Model file for the job. Use its own axes, mm. Face numbers are marked on the shaded views. A direction names the side the tool comes from. Round coordinates to 2 decimals unless told otherwise and drop trailing zeros. Loops run counter-clockwise (first coordinate to the right, second up) from the corner with the lowest first, then second, coordinate; pieces in that order, holes last. Notation, with made-up numbers: M -30.75,-24 L -5.75,-24 A17 ccw -5.75,-8 Z; hole C -31.75,-11 d7. An arc over 180 degrees is marked long. Use a Markdown table: item, result. Add a question column.
Q1. Tool access for the marked faces 1 and 2: list every direction of +Z, -Z, +X, -X, +Y, -Y with a clear straight run to the whole face (end or side of a thin tool).
Q2. Cut at A-A (z = 0). Give the cut face in (x, y), plus the area to 3 significant figures.
Q3. Cut at D-D (y = 9.5). Give the cut face in (x, z), plus the area to 3 significant figures.
Q4. Pin check, flat tips, straight feed: pin 1 (3 mm diameter, centred on x = -1.5, y = 1, fed in from +Z); pin 2 (1.2 mm diameter, centred on y = 1, z = -44.5, fed in from +X); pin 3 (3 mm diameter, centred on x = -1.5, y = 1, fed in from -Z). Stop position of each tip, or through.
Q5. Cut at C-C (x = 48.5). Give the cut face in (y, z).
Q6. Cut at B-B (x = -32). Give the cut face in (y, z), plus the area to 3 significant figures.
Q7. Probe line 1 (Z direction, x = 0, y = 78); line 2 (Y direction, x = -3.5, z = 51); line 3 (Z direction, x = 2, y = 65.5). List the from-to ranges inside material, lowest first. Write a range as from..to.
Autodesk Fusion 360 part; units mm, degrees
sketch "Sketch1" plane through (0, 0, 0) normal (0, 1, 0) x (1, 0, 0)
  line L0 (-3, 15) -> (3, 15)
  line L1 (3, 15) -> (3, 55)
  line L2 (3, 55) -> (-3, 55)
  line L3 (-3, 55) -> (-3, 15)
  line L4 (8.8168, 12.1353) -> (11.2438, 10.3719)
  line L5 (8.8168, 12.1353) -> (6.3897, 13.8986)
  line L6 (6.3897, 13.8986) -> (29.9011, 46.2593)
  line L7 (29.9011, 46.2593) -> (34.7552, 42.7326)
  line L8 (34.7552, 42.7326) -> (11.2438, 10.3719)
  line L9 (14.2658, 4.6353) -> (13.3388, 7.4884)
  line L10 (13.3388, 7.4884) -> (15.1929, 1.7821)
  line L11 (15.1929, 1.7821) -> (53.2352, 14.1428)
  line L12 (53.2352, 14.1428) -> (51.3811, 19.8491)
  line L13 (51.3811, 19.8491) -> (13.3388, 7.4884)
  line L14 (14.2658, -4.6353) -> (13.3388, -7.4884)
  line L15 (13.3388, -7.4884) -> (15.1929, -1.7821)
  line L16 (15.1929, -1.7821) -> (53.2352, -14.1428)
  line L17 (53.2352, -14.1428) -> (51.3811, -19.8491)
  line L18 (51.3811, -19.8491) -> (13.3388, -7.4884)
  line L19 (8.8168, -12.1353) -> (11.2438, -10.3719)
  line L20 (11.2438, -10.3719) -> (34.7552, -42.7326)
  line L21 (34.7552, -42.7326) -> (29.9011, -46.2593)
  line L22 (29.9011, -46.2593) -> (6.3897, -13.8986)
  line L23 (6.3897, -13.8986) -> (8.8168, -12.1353)
  line L24 (0, -15) -> (3, -15)
  line L25 (3, -15) -> (-3, -15)
  line L26 (-3, -15) -> (-3, -55)
  line L27 (-3, -55) -> (3, -55)
  line L28 (3, -55) -> (3, -15)
  line L29 (-8.8168, -12.1353) -> (-6.3897, -13.8986)
  line L30 (-6.3897, -13.8986) -> (-11.2438, -10.3719)
  line L31 (-11.2438, -10.3719) -> (-34.7552, -42.7326)
  line L32 (-34.7552, -42.7326) -> (-29.9011, -46.2593)
  line L33 (-29.9011, -46.2593) -> (-6.3897, -13.8986)
  line L34 (-14.2658, -4.6353) -> (-13.3388, -7.4884)
  line L35 (-13.3388, -7.4884) -> (-15.1929, -1.7821)
  line L36 (-15.1929, -1.7821) -> (-53.2352, -14.1428)
  line L37 (-53.2352, -14.1428) -> (-51.3811, -19.8491)
  line L38 (-51.3811, -19.8491) -> (-13.3388, -7.4884)
  line L39 (-14.2658, 4.6353) -> (-13.3388, 7.4884)
  line L40 (-13.3388, 7.4884) -> (-15.1929, 1.7821)
  line L41 (-15.1929, 1.7821) -> (-53.2352, 14.1428)
  line L42 (-53.2352, 14.1428) -> (-51.3811, 19.8491)
  line L43 (-51.3811, 19.8491) -> (-13.3388, 7.4884)
  line L44 (-8.8168, 12.1353) -> (-6.3897, 13.8986)
  line L45 (-6.3897, 13.8986) -> (-11.2438, 10.3719)
  line L46 (-11.2438, 10.3719) -> (-34.7552, 42.7326)
  line L47 (-34.7552, 42.7326) -> (-29.9011, 46.2593)
  line L48 (-29.9011, 46.2593) -> (-6.3897, 13.8986)
  circle A0 centre (0, 0) radius 60
  dimension "d20" = 15
  dimension "d21" = 15
  dimension "d22" = 15
  dimension "d23" = 15
  dimension "d24" = 15
  dimension "d25" = 15
  dimension "d26" = 15
  dimension "d27" = 15
  dimension "d28" = 15
  dimension "d29" = 40
  dimension "d30" = 6
  dimension "d31" = 40
  dimension "d32" = 3
  dimension "d33" = 3
  dimension "d34" = 40
  dimension "d35" = 6
  dimension "d36" = 3
  dimension "d37" = 6
  dimension "d38" = 40
  dimension "d39" = 6
  dimension "d40" = 3
  dimension "d41" = 40
  dimension "d42" = 6
  dimension "d43" = 3
  dimension "d44" = 40
  dimension "d45" = 6
  dimension "d46" = 40
  dimension "d47" = 3
  dimension "d48" = 6
  dimension "d49" = 40
  dimension "d50" = 6
  dimension "d51" = 3
  dimension "d52" = 6
  dimension "d53" = 40
  dimension "d54" = 6
  dimension "d55" = 3
  dimension "d56" = 6
  dimension "d57" = 40
  dimension "d58" = 6
  dimension "d59" = 3
  dimension "d60" = 6
  dimension "d61" = 40
  dimension "d62" = 6
  dimension "d63" = 3
  dimension "d64" = 6
  dimension "d65" = 40
  dimension "d66" = 6
extrude "Extrude1" add sketch "Sketch1" along normal blind 2.5
sketch "Sketch2" plane through (0, 2.5, 0) normal (0, 1, 0) x (-1, 0, 0)
  line L0 (-11.2438, -10.3719) -> (-6.3897, -13.8986)
  line L1 (-6.3897, -13.8986) -> (-29.9011, -46.2593)
  line L2 (-29.9011, -46.2593) -> (-34.7552, -42.7326)
  line L3 (-34.7552, -42.7326) -> (-11.2438, -10.3719)
  line L4 (-29.9011, 46.2593) -> (-6.3897, 13.8986)
  line L5 (-6.3897, 13.8986) -> (-11.2438, 10.3719)
  line L6 (-11.2438, 10.3719) -> (-34.7552, 42.7326)
  line L7 (-34.7552, 42.7326) -> (-29.9011, 46.2593)
  line L8 (-3, 15) -> (-3, 55)
  line L9 (-3, 55) -> (3, 55)
  line L10 (3, 55) -> (3, 15)
  line L11 (3, 15) -> (-3, 15)
  line L12 (34.7552, -42.7326) -> (29.9011, -46.2593)
  line L13 (29.9011, -46.2593) -> (6.3897, -13.8986)
  line L14 (6.3897, -13.8986) -> (11.2438, -10.3719)
  line L15 (11.2438, -10.3719) -> (34.7552, -42.7326)
  line L16 (3, -15) -> (3, -55)
  line L17 (3, -55) -> (-3, -55)
  line L18 (-3, -55) -> (-3, -15)
  line L19 (-3, -15) -> (3, -15)
  line L20 (13.3388, 7.4884) -> (51.3811, 19.8491)
  line L21 (51.3811, 19.8491) -> (53.2352, 14.1428)
  line L22 (53.2352, 14.1428) -> (15.1929, 1.7821)
  line L23 (15.1929, 1.7821) -> (13.3388, 7.4884)
  line L24 (-13.3388, -7.4884) -> (-51.3811, -19.8491)
  line L25 (-51.3811, -19.8491) -> (-53.2352, -14.1428)
  line L26 (-53.2352, -14.1428) -> (-15.1929, -1.7821)
  line L27 (-15.1929, -1.7821) -> (-13.3388, -7.4884)
  line L28 (6.3897, 13.8986) -> (29.9011, 46.2593)
  line L29 (29.9011, 46.2593) -> (34.7552, 42.7326)
  line L30 (34.7552, 42.7326) -> (11.2438, 10.3719)
  line L31 (11.2438, 10.3719) -> (6.3897, 13.8986)
  line L32 (-53.2352, 14.1428) -> (-51.3811, 19.8491)
  line L33 (-51.3811, 19.8491) -> (-13.3388, 7.4884)
  line L34 (-13.3388, 7.4884) -> (-15.1929, 1.7821)
  line L35 (-15.1929, 1.7821) -> (-53.2352, 14.1428)
  line L36 (53.2352, -14.1428) -> (51.3811, -19.8491)
  line L37 (51.3811, -19.8491) -> (13.3388, -7.4884)
  line L38 (13.3388, -7.4884) -> (15.1929, -1.7821)
  line L39 (15.1929, -1.7821) -> (53.2352, -14.1428)
  circle A0 centre (0, 0) radius 60
  circle A1 centre (0, 0) radius 11
  dimension "d69" = 22
extrude "Extrude2" add sketch "Sketch2" along normal blind 87 contours A1
sketch "Sketch3" plane through (0, 89.5, 0) normal (0, 1, 0) x (-1, 0, 0)
  circle A0 centre (0, 0) radius 11
  arc A1 (-1.2349, 2.288) -> (1.2349, 2.288) centre (0, 0) ccw
  line L0 (1.2349, 2.288) -> (-1.2349, 2.288)
extrude "Extrude3" cut sketch "Sketch3" against normal blind 30 contours A1 L0
extrude "Extrude4" cut 1 faces at (14.2269, 0.8333, -24.6855) along direction (-0.809017, 0, -0.587785) blind 0.25
extrude "Extrude5" cut 1 faces at (-3, 0.8333, -41.6667) along direction (-1, 0, 0) blind 0.25
extrude "Extrude6" cut 1 faces at (-19.081, 0.8333, -21.1588) along direction (-0.809017, 0, 0.587785) blind 0.25
extrude "Extrude7" cut 1 faces at (-27.8737, 0.8333, -5.9023) along direction (-0.309017, 0, 0.951057) blind 0.25
extrude "Extrude8" cut 1 faces at (-38.7003, 0.8333, 15.7289) along direction (0.309017, 0, 0.951057) blind 0.25
extrude "Extrude9" cut 1 faces at (-22.064, 0.8333, 35.4724) along direction (0.809017, 0, 0.587785) blind 0.25
extrude "Extrude10" cut 1 faces at (3, 0.8333, 41.6667) along direction (1, 0, 0) blind 0.25
extrude "Extrude11" cut 1 faces at (19.081, 0.8333, 21.1588) along direction (0.809017, 0, -0.587785) blind 0.25
extrude "Extrude12" cut 1 faces at (27.8737, 0.8333, 5.9023) along direction (0.309017, 0, -0.951057) blind 0.25
extrude "Extrude13" cut 1 faces at (38.7003, 0.8333, -15.7289) along direction (-0.309017, 0, -0.951057) blind 0.25
extrude "Extrude14" cut 1 faces at (27.8737, 0.8333, -5.9023) along direction (0.309017, 0, 0.951057) blind 0.25
extrude "Extrude15" cut 1 faces at (38.7003, 0.8333, 15.7289) along direction (-0.309017, 0, 0.951057) blind 0.25
extrude "Extrude16" cut 1 faces at (22.064, 0.8333, 35.4724) along direction (-0.809017, 0, 0.587785) blind 0.25
extrude "Extrude17" cut 1 faces at (-3, 0.8333, 28.3333) along direction (-1, 0, 0) blind 0.25
extrude "Extrude18" cut 1 faces at (-19.081, 0.8333, 21.1588) along direction (-0.809017, 0, -0.587785) blind 0.25
extrude "Extrude19" cut 1 faces at (-27.8737, 0.8333, 5.9023) along direction (-0.309017, 0, -0.951057) blind 0.25
extrude "Extrude20" cut 1 faces at (-38.7003, 0.8333, -15.7289) along direction (0.309017, 0, -0.951057) blind 0.25
extrude "Extrude21" cut 1 faces at (-22.064, 0.8333, -35.4724) along direction (0.809017, 0, -0.587785) blind 0.25
extrude "Extrude22" cut 1 faces at (3, 0.8333, -28.3333) along direction (1, 0, 0) blind 0.25
extrude "Extrude23" cut 1 faces at (26.9181, 0.8333, -31.9457) along direction (0.809017, 0, 0.587785) blind 0.25
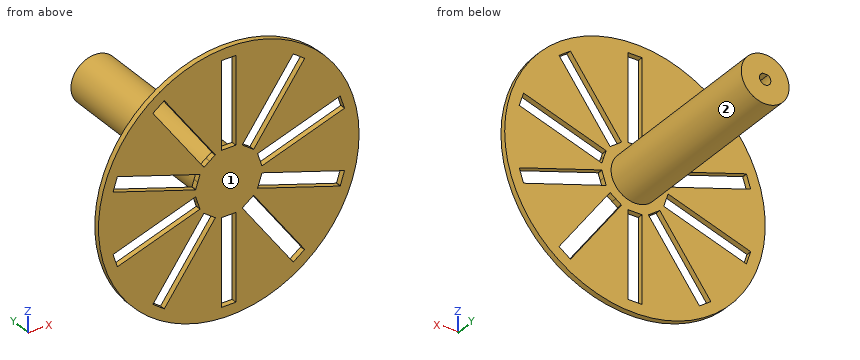
Checked values:
| question | item | result |
|---|---|---|
| 1 | face 1 | +Z, -Z, +X, -X, -Y |
| 1 | face 2 | +Y |
| 2 | outline | M -60,0 L 60,0 L 60,2.5 L 11,2.5 L 11,89.5 L 2.6,89.5 L 2.6,59.5 L -2.6,59.5 L -2.6,89.5 L -11,89.5 L -11,2.5 L -60,2.5 Z |
| 2 | area | 2,060 mm^2 |
| 3 | outline | C 0,0 d22 |
| 3 | area | 380 mm^2 |
| 4 | pin 1 | stops at z = 60 |
| 4 | pin 2 | stops at x = 40.9 |
| 4 | pin 3 | stops at z = -60 |
| 5 | outline | M 0,-35.32 L 2.5,-35.32 L 2.5,-19.18 L 0,-19.18 Z; M 0,-12.34 L 2.5,-12.34 L 2.5,12.34 L 0,12.34 Z; M 0,19.18 L 2.5,19.18 L 2.5,35.32 L 0,35.32 Z |
| 6 | outline | M 0,-50.75 L 2.5,-50.75 L 2.5,-44.73 L 0,-44.73 Z; M 0,-38.52 L 2.5,-38.52 L 2.5,-13.81 L 0,-13.81 Z; M 0,-6.98 L 2.5,-6.98 L 2.5,6.98 L 0,6.98 Z; M 0,13.81 L 2.5,13.81 L 2.5,38.52 L 0,38.52 Z; M 0,44.73 L 2.5,44.73 L 2.5,50.75 L 0,50.75 Z |
| 6 | area | 189 mm^2 |
| 7 | line 1 | z = -11..-2.6, 2.29..11 |
| 7 | line 2 | y = 0..2.5 |
| 7 | line 3 | z = -10.82..-1.66, 1.66..10.82 |
